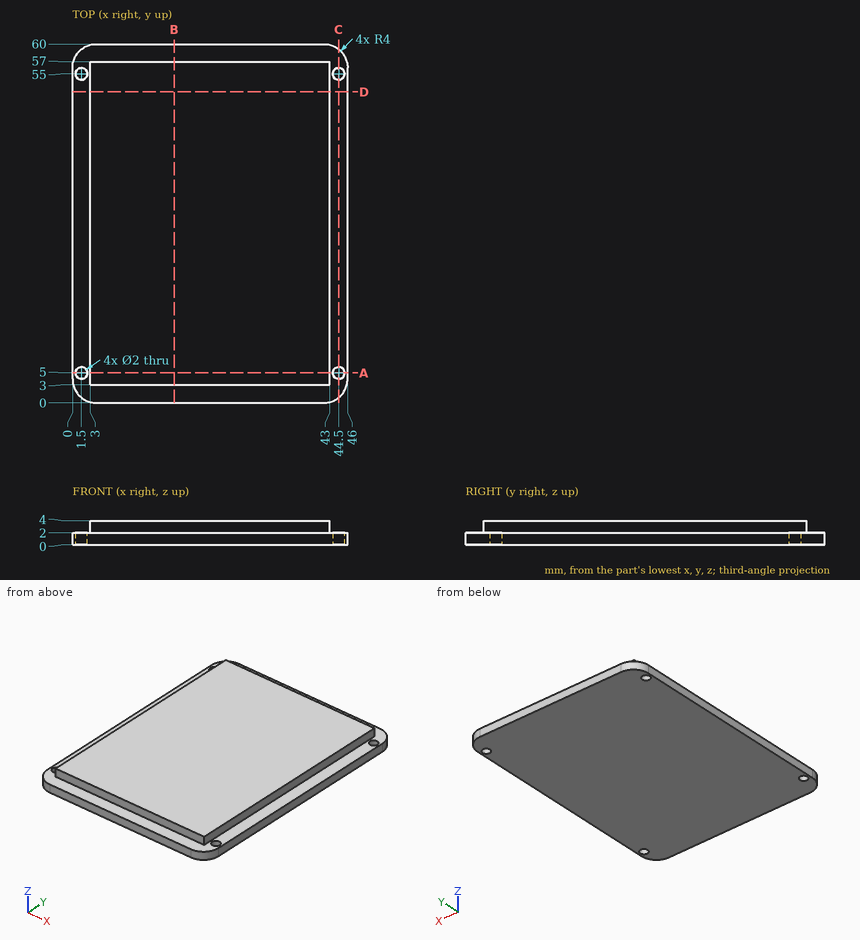
Part print with two shaded views. Sizes in mm from the minimum x, y, z corner. Round coordinates to 2 decimals unless told otherwise and drop trailing zeros. Order: outer loops, then holes, each group sorted by start corner. A loop starts at its lowest first (then second) coordinate and runs counter-clockwise, first axis right, second up. Notation, with made-up numbers: M 51,77 L 94,77 A17 ccw 94,83 Z; hole C -35.5,-30.5 d8. An arc over 180 degrees is marked long. Put each result on its own line as item: value. Start each with the question number.
1. Drill centre lines: probe 1 along X at (y, z) = (55, 1.55); probe 2 along Y at (x, z) = (44.5, 1.35); probe 3 along X at (y, z) = (27, 3.75). Where is each one in solid material? Low to high. Write a range as [from, to].
2. Slice it at B-B on x = 17. List the corners of the cut face in (y, z), then the cut area to 3 significant figures.
3. Slice it at A-A on y = 5. List the corners of the cut face in (x, z), then the cut area to 3 significant figures.
4. Drop flat-ended pins along their axis: pin 1 (2 mm diameter, centred on y = 41.5, z = 2.5, fed in from -X); pin 2 (0.6 mm diameter, centred on y = 17, z = 3.5, fed in from +X); pin 3 (2.5 mm diameter, centred on x = 44.5, y = 55, fed in from +Z); pin 4 (1.2 mm diameter, centred on x = 1.5, y = 5, fed in from -Z). Give the stop position or say it passes through.
5. Slice it at D-D on y = 52. List the corners of the cut face in (x, z), then the cut area to 3 significant figures.
6. Slice it at C-C on x = 44.5. List the corners of the cut face in (y, z), then the cut area to 3 significant figures.
Findings:
1. probe 1: [0, 0.5], [2.5, 43.5], [45.5, 46]
1. probe 2: [0.88, 4], [6, 54], [56, 59.12]
1. probe 3: [3, 43]
2. outline: M 0,0 L 60,0 L 60,2 L 57,2 L 57,4 L 3,4 L 3,2 L 0,2 Z
2. area: 228 mm2
3. outline: M 0,0 L 0.5,0 L 0.5,2 L 0,2 Z; M 2.5,0 L 43.5,0 L 43.5,2 L 43,2 L 43,4 L 3,4 L 3,2 L 2.5,2 Z; M 45.5,0 L 46,0 L 46,2 L 45.5,2 Z
3. area: 164 mm2
4. pin 1: x = 0
4. pin 2: x = 43
4. pin 3: z = 2
4. pin 4: through
5. outline: M 0,0 L 46,0 L 46,2 L 43,2 L 43,4 L 3,4 L 3,2 L 0,2 Z
5. area: 172 mm2
6. outline: M 0.88,0 L 4,0 L 4,2 L 0.88,2 Z; M 6,0 L 54,0 L 54,2 L 6,2 Z; M 56,0 L 59.12,0 L 59.12,2 L 56,2 Z
6. area: 108 mm2
